Source: CAD feature listing. Evaluate the final solid. Frame: model axes, mm. Face numbers are marked on the shaded views. A direction names the side the tool comes from. Coordinates: 2 decimals unless noted, no trailing zeros. Order: outer loops, then holes, each group sorted by start corner. A loop starts at its lowest first (then second) coordinate and runs counter-clockwise, first axis right, second up. Notation, with made-up numbers: (30.25, 23) - (88.25, 23) arc R10 cw to (88.25, 41) - close; hole circle Ø10 at (23, 49.25). An arc over 180 degrees is marked (long way). One line per question, with ' | ' between items.
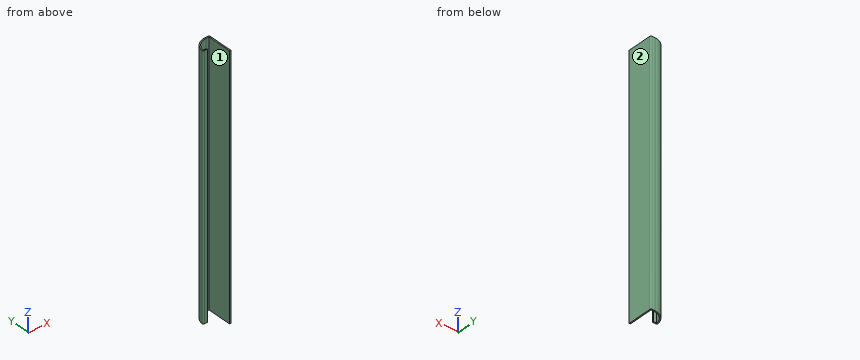
from build123d import *

# Parameters (mm, degrees)
EXTRUDE_THIN1_DEPTH = 190.5
FILLET1_R           = 0.889


with BuildPart() as part:
    # Sketch1 → Extrude-Thin1 (new body)
    with BuildSketch(Plane.XY):
        with BuildLine():
            Line((0, 0), (0, 19.05))
            Line((0, 19.05), (-3.175, 19.05))
            ThreePointArc((-3.175, 19.05), (-9.910192091, 16.260192091), (-12.7, 9.525))
            Line((-12.7, 9.525), (-9.525, 9.525))
            Line((-9.525, 9.525), (-9.525, 10.414))
            Line((-9.525, 10.414), (-11.765120779, 10.414))
            ThreePointArc((-11.765120779, 10.414), (-8.958731149, 15.938185636), (-3.175, 18.161))
            Line((-3.175, 18.161), (-0.889, 18.161))
            Line((-0.889, 18.161), (-0.889, 0))
            Line((-0.889, 0), (0, 0))
        make_face()
    extrude(amount=-EXTRUDE_THIN1_DEPTH)

    # Fillet1
    fillet1_edges = [part.edges().sort_by_distance(p)[0] for p in [
        (-12.7, 9.525, -95.25),
        (0, 19.05, -95.25),
    ]]
    fillet(fillet1_edges, radius=FILLET1_R)


solid = part.part
(1) Material intervals for L1, parallel to Y at x = -3.25, z = -176; L2, parallel to X at y = 13, z = -176.5; L3, parallel to X at y = 3.5, z = -182, sorted ascending. Write a range as from..to.
Taken from the geometry:
L1: y = 18.16..19.05 | L2: x = -12.04..-11.08, -0.89..0 | L3: x = -0.89..0
(2) Cut plane D-D (x = -7.5). Return the cut outline in (y, z), and give its area (3 significant figures).
Taken from the geometry:
outline: (17, -190.5) - (18.01, -190.5) - (18.01, 0) - (17, 0) - close | area: 193 mm²
(3) Pin query (flat end, axial travel): P1, Ø4, axis at y = 14.5, z = -79.5, coming from the -X side; P2, Ø3, axis at x = -6.5, z = -95, coming from the -Y side; P3, Ø4, axis at y = 16.5, z = -42.5, coming from the -X side. Return the tip coordinate at first contact, or that it passes through.
Taken from the geometry:
P1: stops at x = -12.22 | P2: stops at y = 16.69 | P3: stops at x = -11.3
(4) Cut plane C-C (y = 1.75). Return the cut outline in (x, z).
Taken from the geometry:
outline: (-0.89, -190.5) - (0, -190.5) - (0, 0) - (-0.89, 0) - close
(5) Cut plane B-B (z = -178). Return the cut outline in (x, y) (3 decimals), and give its area (3 significant figures).
Taken from the geometry:
outline: (-12.649, 10.506) arc R0.889 ccw to (-11.765, 9.525) - (-9.525, 9.525) - (-9.525, 10.414) - (-11.765, 10.414) arc R8.636 cw to (-3.175, 18.161) - (-0.889, 18.161) - (-0.889, 0) - (0, 0) - (0, 18.161) arc R0.889 ccw to (-0.889, 19.05) - (-3.175, 19.05) arc R9.525 ccw to start | area: 33.3 mm²
(6) Set-up query: the marked faces 1 and 2. Return all of +Z, -Z, +X, -X, +Y, -Y with unobstructed straight access to the full face (end or side cutting, diameter ignored); none if empty.
Taken from the geometry:
face 1: +Z, -Z, -Y | face 2: +Z, -Z, +X, +Y, -Y
(7) Cut plane A-A (y = 14). Return the cut outline in (x, z).
Taken from the geometry:
outline: (-11.58, -190.5) - (-10.56, -190.5) - (-10.56, 0) - (-11.58, 0) - close; (-0.89, -190.5) - (0, -190.5) - (0, 0) - (-0.89, 0) - close
